```python
from build123d import *

# Parameters (mm, degrees)
SKETCH_1_W             = 40
SKETCH_1_H             = 40
EXTRUDE_1_DEPTH        = 20
FILLET_START           = -15
FILLET_1_OUTLINE_W     = 42
FILLET_1_OUTLINE_H     = 6
FILLET_1_DEPTH         = 2.272077939
FILLET_START_2         = 26.870057685
FILLET_2_OUTLINE_W     = 42
FILLET_2_OUTLINE_H     = 6
FILLET_2_DEPTH         = 2.129942315
SKETCH_2_W             = 40
SKETCH_2_H             = 20
SKETCH_2_W_2           = 34
SKETCH_2_H_2           = 18
CUT_EXTRUDE_1_DEPTH    = 2
FILLET_1_2_R           = 1
FILLET_2_2_R           = 1
FILLET_3_R             = 1
FILLET_4_R             = 1
SKETCH_3_R             = 5
EXTRUDE_2_DEPTH        = 7
SKETCH_4_R             = 12
EXTRUDE_3_DEPTH        = 2
CUT_EXTRUDE_2_REACH    = 59.315
SKETCH_5_R             = 1.5
SKETCH_6_W             = 4
SKETCH_6_H             = 20
EXTRUDE_4_DEPTH        = 8
CUT_EXTRUDE_3_REACH    = 49.875
SKETCH_7_R             = 2
FILLET_5_R             = 2
FILLET_6_R             = 2
FILLET_5_OF_MIRROR_1_R = 2
FILLET_6_OF_MIRROR_1_R = 2


with BuildPart() as part:
    # Sketch 1 → Extrude 1 (new body)
    with BuildSketch(Plane(origin=(0, 0, 0), x_dir=(1, 0, 0), z_dir=(0, 1, 0))):
        Rectangle(SKETCH_1_W, SKETCH_1_H)
    extrude(amount=EXTRUDE_1_DEPTH)

    # Fillet 1: read off the stored shape, not the designer's step
    # Fillet 1 outline → Fillet 1 (cut)
    with BuildSketch(Plane(origin=(0, 0, 0), x_dir=(1, 0, 0), z_dir=(0, 0.707106781186547, -0.707106781186548)).offset(FILLET_START)):
        with Locations((0, -14)):
            Rectangle(FILLET_1_OUTLINE_W, FILLET_1_OUTLINE_H)
    extrude(amount=FILLET_1_DEPTH, mode=Mode.SUBTRACT)

    # Fillet 2: read off the stored shape, not the designer's step
    # Fillet 2 outline → Fillet 2 (cut)
    with BuildSketch(Plane(origin=(0, 0, 0), x_dir=(1, 0, 0), z_dir=(0, 0.707106781186547, 0.707106781186548)).offset(FILLET_START_2)):
        Rectangle(FILLET_2_OUTLINE_W, FILLET_2_OUTLINE_H)
    extrude(amount=FILLET_2_DEPTH, mode=Mode.SUBTRACT)

    # Sketch 2 → Cut-Extrude 1 (cut)
    with BuildSketch(Plane(origin=(0, 0, -20), x_dir=(-1, 0, 0), z_dir=(0, 0, -1))):
        with Locations((0, 10)):
            Rectangle(SKETCH_2_W, SKETCH_2_H)
        with Locations((2, 10)):
            Rectangle(SKETCH_2_W_2, SKETCH_2_H_2, mode=Mode.SUBTRACT)
    extrude(amount=-CUT_EXTRUDE_1_DEPTH, mode=Mode.SUBTRACT)

    # Fillet 1 2
    fillet_1_2_edges = [part.edges().sort_by_distance(p)[0] for p in [
        (15, 1, -19),
    ]]
    fillet(fillet_1_2_edges, radius=FILLET_1_2_R)

    # Fillet 2 2
    fillet_2_2_edges = [part.edges().sort_by_distance(p)[0] for p in [
        (15, 19, -19),
    ]]
    fillet(fillet_2_2_edges, radius=FILLET_2_2_R)

    # Fillet 3
    fillet_3_edges = [part.edges().sort_by_distance(p)[0] for p in [
        (-19, 1, -19),
    ]]
    fillet(fillet_3_edges, radius=FILLET_3_R)

    # Fillet 4
    fillet_4_edges = [part.edges().sort_by_distance(p)[0] for p in [
        (-19, 19, -19),
    ]]
    fillet(fillet_4_edges, radius=FILLET_4_R)

    # Sketch 3 → Extrude 2 (add)
    with BuildSketch(Plane(origin=(0, 0, -20), x_dir=(-1, 0, 0), z_dir=(0, 0, -1))):
        with Locations(Location((8, 10, 0), (0, 0, 180))):
            Circle(SKETCH_3_R)
    extrude(amount=EXTRUDE_2_DEPTH)

    # Sketch 4 → Extrude 3 (add)
    with BuildSketch(Plane(origin=(0, 0, -27), x_dir=(-1, 0, 0), z_dir=(0, 0, -1))):
        with Locations((8, 10)):
            Circle(SKETCH_4_R)
    extrude(amount=EXTRUDE_3_DEPTH)

    # Sketch 5 → Cut-Extrude 2 (cut, up to next)
    with BuildSketch(Plane(origin=(0, 0, -29), x_dir=(-1, 0, 0), z_dir=(0, 0, -1)), mode=Mode.PRIVATE) as cut_extrude_2_sk1:
        with Locations((8, 17)):
            Circle(SKETCH_5_R)
    cut_extrude_2_tool1 = extrude(cut_extrude_2_sk1.sketch, amount=-CUT_EXTRUDE_2_REACH, mode=Mode.PRIVATE) & part.part
    # Sketch 5 → Cut-Extrude 2 (cut, up to next)
    with BuildSketch(Plane(origin=(0, 0, -29), x_dir=(-1, 0, 0), z_dir=(0, 0, -1)), mode=Mode.PRIVATE) as cut_extrude_2_sk2:
        with Locations((15, 10)):
            Circle(SKETCH_5_R)
    cut_extrude_2_tool2 = extrude(cut_extrude_2_sk2.sketch, amount=-CUT_EXTRUDE_2_REACH, mode=Mode.PRIVATE) & part.part
    # Sketch 5 → Cut-Extrude 2 (cut, up to next)
    with BuildSketch(Plane(origin=(0, 0, -29), x_dir=(-1, 0, 0), z_dir=(0, 0, -1)), mode=Mode.PRIVATE) as cut_extrude_2_sk3:
        with Locations((8, 3)):
            Circle(SKETCH_5_R)
    cut_extrude_2_tool3 = extrude(cut_extrude_2_sk3.sketch, amount=-CUT_EXTRUDE_2_REACH, mode=Mode.PRIVATE) & part.part
    # Sketch 5 → Cut-Extrude 2 (cut, up to next)
    with BuildSketch(Plane(origin=(0, 0, -29), x_dir=(-1, 0, 0), z_dir=(0, 0, -1)), mode=Mode.PRIVATE) as cut_extrude_2_sk4:
        with Locations((1, 10)):
            Circle(SKETCH_5_R)
    cut_extrude_2_tool4 = extrude(cut_extrude_2_sk4.sketch, amount=-CUT_EXTRUDE_2_REACH, mode=Mode.PRIVATE) & part.part
    add(cut_extrude_2_tool1.solids().sort_by_distance((-8, 17, -29))[0], mode=Mode.SUBTRACT)
    add(cut_extrude_2_tool2.solids().sort_by_distance((-15, 10, -29))[0], mode=Mode.SUBTRACT)
    add(cut_extrude_2_tool3.solids().sort_by_distance((-8, 3, -29))[0], mode=Mode.SUBTRACT)
    add(cut_extrude_2_tool4.solids().sort_by_distance((-1, 10, -29))[0], mode=Mode.SUBTRACT)

    # Sketch 6 → Extrude 4 (add)
    with BuildSketch(Plane.ZY.offset(20)):
        with Locations((-10, 10)):
            Rectangle(SKETCH_6_W, SKETCH_6_H)
    extrude_4 = extrude(amount=EXTRUDE_4_DEPTH)

    # Sketch 7 → Cut-Extrude 3 (cut, up to next)
    with BuildSketch(Plane(origin=(0, 0, -12), x_dir=(-1, 0, 0), z_dir=(0, 0, -1)), mode=Mode.PRIVATE) as cut_extrude_3_sk1:
        with Locations((24, 15)):
            Circle(SKETCH_7_R)
    cut_extrude_3_tool1 = extrude(cut_extrude_3_sk1.sketch, amount=-CUT_EXTRUDE_3_REACH, mode=Mode.PRIVATE) & part.part
    # Sketch 7 → Cut-Extrude 3 (cut, up to next)
    with BuildSketch(Plane(origin=(0, 0, -12), x_dir=(-1, 0, 0), z_dir=(0, 0, -1)), mode=Mode.PRIVATE) as cut_extrude_3_sk2:
        with Locations((24, 5)):
            Circle(SKETCH_7_R)
    cut_extrude_3_tool2 = extrude(cut_extrude_3_sk2.sketch, amount=-CUT_EXTRUDE_3_REACH, mode=Mode.PRIVATE) & part.part
    cut_extrude_3_1 = cut_extrude_3_tool1.solids().sort_by_distance((-24, 15, -12))[0]
    add(cut_extrude_3_1, mode=Mode.SUBTRACT)
    cut_extrude_3_2 = cut_extrude_3_tool2.solids().sort_by_distance((-24, 5, -12))[0]
    add(cut_extrude_3_2, mode=Mode.SUBTRACT)
    cut_extrude_3 = cut_extrude_3_1 + cut_extrude_3_2  # Cut-Extrude 3 as one shape, for the pattern or mirror that repeats it

    # Fillet 5
    fillet_5_edges = [part.edges().sort_by_distance(p)[0] for p in [
        (-28, 20, -10),
    ]]
    fillet(fillet_5_edges, radius=FILLET_5_R)

    # Fillet 6
    fillet_6_edges = [part.edges().sort_by_distance(p)[0] for p in [
        (-28, 0, -10),
    ]]
    fillet(fillet_6_edges, radius=FILLET_6_R)

    # Mirror 1: Extrude 4, Cut-Extrude 3 across plane
    add(extrude_4.mirror(Plane(origin=(0, 0, 0), x_dir=(0, 0, 1), z_dir=(1, 0, 0))))
    add(cut_extrude_3.mirror(Plane(origin=(0, 0, 0), x_dir=(0, 0, 1), z_dir=(1, 0, 0))), mode=Mode.SUBTRACT)

    # Fillet 5 of Mirror 1
    fillet_5_of_mirror_1_edges = [part.edges().sort_by_distance(p)[0] for p in [
        (28, 20, -10),
    ]]
    fillet(fillet_5_of_mirror_1_edges, radius=FILLET_5_OF_MIRROR_1_R)

    # Fillet 6 of Mirror 1
    fillet_6_of_mirror_1_edges = [part.edges().sort_by_distance(p)[0] for p in [
        (28, 0, -10),
    ]]
    fillet(fillet_6_of_mirror_1_edges, radius=FILLET_6_OF_MIRROR_1_R)


solid = part.part
```
Verification items for the finished model (mm, model axes). A direction names the side the tool comes from. Coordinates: 2 decimals unless noted, no trailing zeros. Write each loop counter-clockwise with the first axis right and the second up, starting at its lowest first coordinate (ties: lowest second). Pieces come first, ordered by that corner, then holes. Notation, with made-up numbers: M 16,31 L 70,31 A20 ccw 70,45 Z; hole C 35,11.25 d5. An arc over 180 degrees is marked long. One line per item, written item: value.
Item 1: Section check D-D, the plane z = -14. Record the boundary of the cut face in (x, y), plus the area to 3 significant figures.
Check sheet entries:
outline: M -20,0 L 20,0 L 20,20 L -20,20 Z
area: 800 mm^2
Item 2: Access from +Z, -Z, +X, -X, +Y, -Y to the whole of each face (thin tool, end or side, straight path). Record for faces 4 (the flat face through (-19, 10, -19)), 5 (the flat face through (20, 10, -15)), 6 (the flat face through (-24, 10, -8)), 7 (the flat face through (-24, 10, -12)), 8 (the cylindrical face through (-6.8, 2.1, -28)).
Check sheet entries:
face 4: -X, +Y, -Y
face 5: -Z, +X, +Y, -Y
face 6: +Z, -X, +Y, -Y
face 7: -Z, -X, +Y, -Y
face 8: -Z
Item 3: Section check B-B, the plane y = 14.25. State how many separate pieces and enclosed holes the cut face has, plus the area to 3 significant figures.
Check sheet entries:
separate pieces: 3
enclosed holes: 0
area: 1,700 mm^2
Item 4: Gauge pin test, flat ends, axial feed: pin 1 Ø5 at (x, y) = (-24, 15) entering from -Z; pin 2 Ø1.5 at (x, z) = (-14.5, -11.5) entering from +Y; pin 3 Ø6.5 at (y, z) = (12, -16) entering from +X. Record the tip position at first contact, or that the pin passes through.
Check sheet entries:
pin 1: stops at z = -12
pin 2: stops at y = 20
pin 3: stops at x = 20
Item 5: Section check C-C, the plane x = 7.5. Record the boundary of the cut face in (y, z).
Check sheet entries:
outline: M 0,-18 L 1,-18 L 1,-20 L 19,-20 L 19,-18 L 20,-18 L 20,18 L 18,20 L 2,20 L 0,18 Z
Item 6: Mould release check, pull along Y, two halves, no side actions. Record for faces 1 (the cylindrical face through (-22, 5, -10)), 2 (the flat face through (24, 10, -12)), 3 (the cylindrical face through (27.43, 0.6, -9.97)): pulls with the +Y half, pulls with the -Y half, needs draft (parallel to the pull), parting line crosses it, or undercut.
Check sheet entries:
face 1: undercut
face 2: needs draft
face 3: pulls with the -Y half
Item 7: Section check A-A, the plane x = -8. Record the boundary of the cut face in (y, z), plus the area to 3 significant figures.
Check sheet entries:
outline: M -2,-29 L 1.5,-29 L 1.5,-27 L -2,-27 Z; M 0,-18 L 1,-18 L 1,-20 L 5,-20 L 5,-27 L 4.5,-27 L 4.5,-29 L 15.5,-29 L 15.5,-27 L 15,-27 L 15,-20 L 19,-20 L 19,-18 L 20,-18 L 20,18 L 18,20 L 2,20 L 0,18 Z; M 18.5,-29 L 22,-29 L 22,-27 L 18.5,-27 Z
area: 898 mm^2
Item 8: Scan lines: line 1 along Y through (x, z) = (24, -10); line 2 along Y through (x, z) = (-8, -28.3); line 3 along Z through (x, y) = (-14.5, 8.5). Record each from-to range of solid material in increasing order.
Check sheet entries:
line 1: y = 0 to 3, 7 to 13, 17 to 20
line 2: y = -2 to 1.5, 4.5 to 15.5, 18.5 to 22
line 3: z = -29 to -27, -20 to 20
